```python
from build123d import *

# Parameters (mm, degrees)
SKETCH1_W           = 3.2
SKETCH1_H           = 10
BOSS_EXTRUDE1_DEPTH = 3.2


with BuildPart() as part:
    # Sketch1 → Boss-Extrude1 (new body)
    with BuildSketch(Plane(origin=(0, 0, 0), x_dir=(1, 0, 0), z_dir=(0, 1, 0))):
        with BuildLine():
            Line((-87.5, 7.5), (-87.5, 20))
            Line((-87.5, 20), (-84.3, 20))
            Line((-84.3, 20), (-84.3, 35))
            Line((-84.3, 35), (-87.5, 35))
            Line((-87.5, 35), (-87.5, 50))
            Line((-87.5, 50), (-70, 50))
            Line((-70, 50), (-70, 46.8))
            Line((-70, 46.8), (-50, 46.8))
            Line((-50, 46.8), (-50, 50))
            Line((-50, 50), (-30, 50))
            Line((-30, 50), (-30, 46.8))
            Line((-30, 46.8), (-10, 46.8))
            Line((-10, 46.8), (-10, 50))
            Line((-10, 50), (10, 50))
            Line((10, 50), (10, 46.8))
            Line((10, 46.8), (30, 46.8))
            Line((30, 46.8), (30, 50))
            Line((30, 50), (50, 50))
            Line((50, 50), (50, 46.8))
            Line((50, 46.8), (70, 46.8))
            Line((70, 46.8), (70, 50))
            Line((70, 50), (87.5, 50))
            Line((87.5, 50), (87.5, 35))
            Line((87.5, 35), (84.3, 35))
            Line((84.3, 35), (84.3, 20))
            Line((84.3, 20), (87.5, 20))
            Line((87.5, 20), (87.5, 7.5))
            Line((87.5, 7.5), (84.3, 7.5))
            ThreePointArc((84.3, 7.5), (76.8, 0), (84.3, -7.5))
            Line((84.3, -7.5), (87.5, -7.5))
            Line((87.5, -7.5), (87.5, -20))
            Line((87.5, -20), (84.3, -20))
            Line((84.3, -20), (84.3, -35))
            Line((84.3, -35), (87.5, -35))
            Line((87.5, -35), (87.5, -50))
            Line((87.5, -50), (70, -50))
            Line((70, -50), (70, -46.8))
            Line((70, -46.8), (50, -46.8))
            Line((50, -46.8), (50, -50))
            Line((50, -50), (30, -50))
            Line((30, -50), (30, -46.8))
            Line((30, -46.8), (10, -46.8))
            Line((10, -46.8), (10, -50))
            Line((10, -50), (-10, -50))
            Line((-10, -50), (-10, -46.8))
            Line((-10, -46.8), (-30, -46.8))
            Line((-30, -46.8), (-30, -50))
            Line((-30, -50), (-50, -50))
            Line((-50, -50), (-50, -46.8))
            Line((-50, -46.8), (-70, -46.8))
            Line((-70, -46.8), (-70, -50))
            Line((-70, -50), (-87.5, -50))
            Line((-87.5, -50), (-87.5, -35))
            Line((-87.5, -35), (-84.3, -35))
            Line((-84.3, -35), (-84.3, -20))
            Line((-84.3, -20), (-87.5, -20))
            Line((-87.5, -20), (-87.5, -7.5))
            Line((-87.5, -7.5), (-84.3, -7.5))
            Line((-84.3, -7.5), (-84.3, 7.5))
            Line((-84.3, 7.5), (-87.5, 7.5))
        make_face()
        with Locations((-77.7, 35)):
            Rectangle(SKETCH1_W, SKETCH1_H, mode=Mode.SUBTRACT)
        with Locations((-77.7, -35)):
            Rectangle(SKETCH1_W, SKETCH1_H, mode=Mode.SUBTRACT)
    extrude(amount=BOSS_EXTRUDE1_DEPTH)


solid = part.part
```
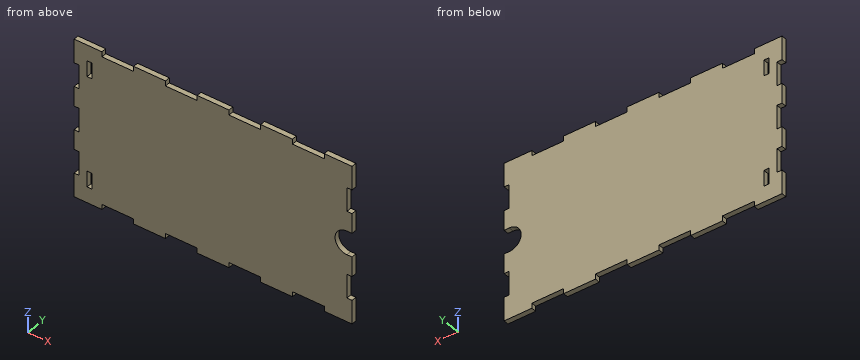
Here's how the part is built. I have some questions about the finished solid (model axes, mm). Coordinates: 2 decimals unless noted, no trailing zeros. Order: outer loops, then holes, each group sorted by start corner. A loop starts at its lowest first (then second) coordinate and runs counter-clockwise, first axis right, second up. Notation, with made-up numbers: (51, 18) -> (62, 18) arc R26 cw to (62, 39) -> close; hole circle Ø3 at (13, -25). An arc over 180 degrees is marked (long way). Return JSON: item names as keys, results as strings.
1) If I drill on probe 1 along X at (y, z) = (1.45, 31.5); probe 2 along X at (y, z) = (2.6, -35.5); probe 3 along X at (y, z) = (1.75, 29.5), over which ranges is the centre line in solid material (lowest first)?
Conclusion:
{"probe 1": "x = -84.3 to -79.3, -76.1 to 84.3", "probe 2": "x = -87.5 to -79.3, -76.1 to 87.5", "probe 3": "x = -84.3 to 84.3"}
2) If we section it at A-A on y = 1.05: State how many separate pieces and enclosed holes the cut face has, plus the area to 3 significant figures.
Conclusion:
{"separate pieces": "1", "enclosed holes": "2", "area": "16,500 mm²"}
3) I'm going to push flat-ended pins straight in: P1, Ø1, axis at y = 2, z = -31, coming from the -X side; P2, Ø1, axis at y = 2, z = -29, coming from the +X side; P3, Ø1, axis at x = -57, y = 2, coming from the -Z side. Where does each tip first touch, or does it pass through?
Conclusion:
{"P1": "stops at x = -84.3", "P2": "stops at x = 84.3", "P3": "stops at z = -46.8"}
4) If we section it at C-C on z = -4.5: List the corners of the cut face in (x, y) for me.
Conclusion:
{"outline": "(-84.3, 0) -> (78.3, 0) -> (78.3, 3.2) -> (-84.3, 3.2) -> close"}
5) If we section it at B-B on x = -25: List the corners of the cut face in (y, z) for me, plus the area to 3 significant figures.
Conclusion:
{"outline": "(0, -46.8) -> (3.2, -46.8) -> (3.2, 46.8) -> (0, 46.8) -> close", "area": "300 mm²"}
